Autodesk Fusion 360 part; units mm, degrees
sketch "Sketch1" plane through (0, 0, 0) normal (0, 0, 1) x (1, 0, 0)
  line L0 (0, 0) -> (0, 31.8988)
  line L1 (0, 31.8988) -> (70, 31.8988)
  line L2 (0, 0) -> (0, -30)
  line L3 (0, -30) -> (70, -30)
  arc A0 (70, -30) -> (70, 31.8988) centre (70, 0.9494) ccw
  dimension "d1" = 70
  dimension "d2" = 30
  dimension "d23" = 70
extrude "Extrude1" add sketch "Sketch1" along normal mid plane 100
sketch "Sketch6" plane through (0, 0, 0) normal (0, 0, 1) x (1, 0, 0)
  line L0 (0, 0) -> (0, 40)
  line L1 (0, 0) -> (0, -40)
  line L2 (0, 40) -> (-80, 40)
  line L3 (-80, -40) -> (0, -40)
  line L4 (-80, -40) -> (-80, 40) construction
  arc A0 (-80, 40) -> (-80, -40) centre (-80, 0) ccw
  dimension "d24" = 40
  dimension "d25" = 40
  dimension "d42" = 80
extrude "Extrude5" add sketch "Sketch6" along normal mid plane 140
sketch "Sketch8" plane through (0, 0, 70) normal (0, 0, 1) x (-1, 0, 0)
  line L0 (0, 40) -> (0, -40)
  line L1 (0, -40) -> (80, -40)
  line L2 (80, 40) -> (0, 40)
  circle A0 centre (80, 0) radius 17.5 construction
  line L3 (80, 0) -> (80, -30) construction
  line L4 (80, 0) -> (48.1334, 0) construction
  line L5 (80, 0) -> (53.2858, -26.7142) construction
  circle A1 centre (67.6256, -12.3744) radius 2
  circle A2 centre (92.3744, -12.3744) radius 2
  circle A3 centre (92.3744, 12.3744) radius 2
  circle A4 centre (67.6256, 12.3744) radius 2
  arc A5 (80, -40) -> (80, 40) centre (80, 0) ccw
  dimension "d33" = 35
  dimension "d35" = 45
  dimension "d36" = 4
  dimension "d38" = 360
sketch "Sketch9" plane through (0, -40, 0) normal (0, -1, 0) x (1, 0, 0)
  line L0 (0, -70) -> (0, 70)
  line L1 (0, 70) -> (-80, 70)
  line L2 (-80, 70) -> (-80, -70)
  line L3 (-80, -70) -> (0, -70)
  line L4 (-160, 55) -> (-20, 55)
  line L5 (-20, 55) -> (-20, -55)
  line L6 (-20, -55) -> (-160, -55)
  line L7 (-160, -55) -> (-160, 55)
  dimension "d44" = 15
  dimension "d45" = 15
  dimension "d46" = 20
extrude "Extrude8" cut sketch "Sketch9" against normal blind 140 contours L2 L4 L6 L7 | L2 L4 L5 L6
sketch "Sketch10" plane through (0, 0, 0) normal (0, 1, 0) x (1, 0, 0)
  line L0 (70, -35) -> (70, -15) construction
  line L1 (70, 15) -> (70, 35) construction
  line L2 (70, 50) -> (70, -50)
  point P0 (70, -50)
  point P1 (70, 50)
  dimension "d49" = 20
  dimension "d50" = 20
  dimension "d51" = 30
  dimension "d52" = 15
  dimension "d53" = 15
scale "Scale1" factor 0.5 about (0, 40, 70) bodies 1
Part model, mm, in its own coordinate system. A direction names the side the tool comes from. Round coordinates to 2 decimals unless told otherwise and drop trailing zeros. Write each loop counter-clockwise with the first axis right and the second up, starting at its lowest first coordinate (ties: lowest second). Pieces come first, ordered by that corner, then holes. Notation, with made-up numbers: M 7.5,17.25 L 33.5,17.25 A28 ccw 33.5,37.25 Z; hole C 2.5,49.25 d2. An arc over 180 degrees is marked long. Return JSON: item names as keys, results as strings. Group by question number.
(1) Saw through at A-A on z = 21.5. Write the cut outline in (x, y).
(2) Two-plate mould, pull along Z, no slides. Class faces 5 (the face through (-35, 20, 62.5)), 6 (the face through (25, 21, 60)), 7 (the face through (-6, 40, 35)): +Z half, -Z half, draft (parallel to the pull), parting line (faces both ways), or undercut.
(3) Pin check, flat tips, straight feed: pin 1 Ø2 at (x, y) = (28.5, 31.5) entering from -Z; pin 2 Ø2 at (x, y) = (20.5, 11.5) entering from +Z; pin 3 Ø3 at (x, z) = (6.5, 26) entering from +Y. Stop position of each tip, or through.
(4) Drill centre lines: probe 1 along Z at (x, y) = (-18, 7); probe 2 along X at (y, z) = (38, 61.5); probe 3 along Z at (x, y) = (29.5, 35). Where is each one in solid material? Low to high.
(5) Which spindle directions (+Z, -Z, +X, -X, +Y, -Y) get a long thin tool onto all of the face, cutting with end or side? Do faces 1 (the face through (17, 5, 35)), 2 (the face through (-35, 20, 7.5)), 3 (the face through (25, 21, 10)), 4 (the face through (17, 35.949, 35)). Say none if no direction does.
(6) Saw through at B-B on y = 20. Write the cut outline in (x, z), then the cut area to 3 significant figures.
(7) Saw through at C-C on x = 27.5. Write the cut outline in (y, z), then the cut area to 3 significant figures.
(8) Saw through at D-D on y = 12. Write the cut outline in (x, z).
Returned:
{
 "1": {"outline": "M -10,0 L 0,0 L 0,5 L 35,5 A15.47 ccw 35,35.95 L 0,35.95 L 0,40 L -10,40 Z"},
 "2": {"face 5": "undercut", "face 6": "+Z half", "face 7": "draft"},
 "3": {"pin 1": "z = 10", "pin 2": "z = 60", "pin 3": "y = 35.95"},
 "4": {"probe 1": "0 to 7.5, 62.5 to 70", "probe 2": "-10 to 0", "probe 3": "10 to 60"},
 "5": {"face 1": "+Z, -Z, +X, -Y", "face 2": "-X, +Y, -Y", "face 3": "-Z, +X, +Y, -Y", "face 4": "+Z, -Z, +X, +Y"},
 "6": {"outline": "M -60,0 L 0,0 L 0,10 L 50.47,10 L 50.47,60 L 0,60 L 0,70 L -60,70 L -60,62.5 L -10,62.5 L -10,7.5 L -60,7.5 Z", "area": "3,970 mm²"},
 "7": {"outline": "M 5,10 L 35.95,10 L 35.95,60 L 5,60 Z", "area": "1,550 mm²"},
 "8": {"outline": "M -58.33,0 L 0,0 L 0,10 L 47.95,10 L 47.95,60 L 0,60 L 0,70 L -58.33,70 L -58.33,62.5 L -10,62.5 L -10,7.5 L -58.33,7.5 Z"}
}
